Verification items for the finished model (mm, model axes). Face numbers are marked on the shaded views. A direction names the side the tool comes from. Give positions to 0.01 mm unless a question says otherwise; leave off trailing zeros. Loops run counter-clockwise (first coordinate to the right, second up) from the corner with the lowest first, then second, coordinate; pieces in that order, holes last. Notation, with made-up numbers: M 51,37.25 L 92,37.25 A35 ccw 92,70.25 Z; hole C 56.5,31 d1. An arc over 180 degrees is marked long. Answer in a Markdown table with one row per item.
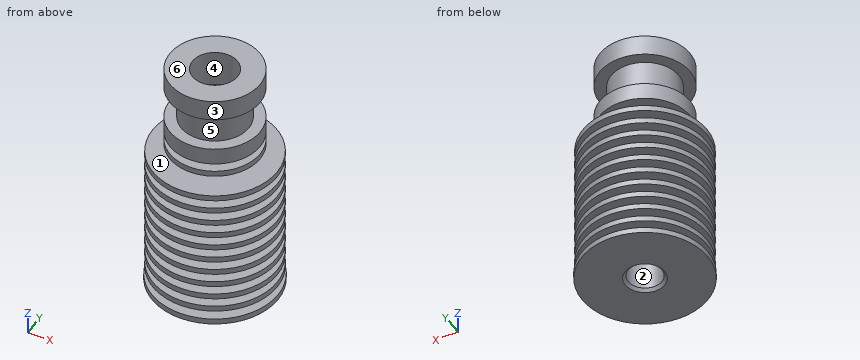
```python
from build123d import *

# Parameters (mm, degrees)
F2_W           = 5
F2_H           = 6
F2_H_2         = 1.5
F4_W           = 8
F4_H           = 1.5
F4_W_2         = 8.1
F4_W_3         = 8.2
F4_W_4         = 8.3
F4_W_5         = 8.4
F4_W_6         = 8.5
F4_W_7         = 8.6
F4_W_8         = 8.7
F4_W_9         = 8.8
F4_W_10        = 8.9
F9_D           = 6
F9_DEPTH       = 10
F9_CSINK_D     = 7
F9_CSINK_ANGLE = 90


with BuildPart() as f1:
    # F0 (on Front) → F1 (revolve)
    with BuildSketch(Plane.XZ):
        Polygon((0, 42.7), (0, 0), (11.15, 0), (11.15, 1), (11, 1), (11, 26), (8, 26), (8, 42.7), align=None)
    revolve(axis=Axis((0, 0, 21.35), (0, 0, 1)))

    # F2 (on Front) → F3 (revolve, cut)
    with BuildSketch(Plane.XZ):
        with Locations((8.5, 36)):
            Rectangle(F2_W, F2_H)
        with Locations((8.5, 29.25)):
            Rectangle(F2_W, F2_H_2)
        with Locations((8.5, 26.75)):
            Rectangle(F2_W, F2_H_2)
    revolve(axis=Axis((0, 0, 22.5), (0, 0, 1)), mode=Mode.SUBTRACT)

    # F4 (on Front) → F5 (revolve, cut)
    with BuildSketch(Plane.XZ):
        with Locations((11, 1.75)):
            Rectangle(F4_W, F4_H)
        with Locations((10.95, 4.25)):
            Rectangle(F4_W_2, F4_H)
        with Locations((10.9, 6.75)):
            Rectangle(F4_W_3, F4_H)
        with Locations((10.85, 9.25)):
            Rectangle(F4_W_4, F4_H)
        with Locations((10.8, 11.75)):
            Rectangle(F4_W_5, F4_H)
        with Locations((10.75, 14.25)):
            Rectangle(F4_W_6, F4_H)
        with Locations((10.7, 16.75)):
            Rectangle(F4_W_7, F4_H)
        with Locations((10.65, 19.25)):
            Rectangle(F4_W_8, F4_H)
        with Locations((10.6, 21.75)):
            Rectangle(F4_W_9, F4_H)
        with Locations((10.55, 24.25)):
            Rectangle(F4_W_10, F4_H)
    revolve(axis=Axis((0, 0, 13.092068), (0, 0, 1)), mode=Mode.SUBTRACT)

    # F6 (on Front) → F7 (revolve, cut)
    with BuildSketch(Plane.XZ):
        Polygon((0, 42.7), (0, 0), (3, 0), (3, 15.1), (2.1, 15.640775), (2.1, 35.058365), (4, 36.2), (4, 42.7), align=None)
    revolve(axis=Axis((0, 0, 21.35), (0, 0, 1)), mode=Mode.SUBTRACT)

    # F9
    with Locations(Plane(origin=(0, 0, 0), x_dir=(1, 0, 0), z_dir=(0, 0, -1))):
        with Locations((0, 0)):
            CounterSinkHole(F9_D / 2, F9_CSINK_D / 2, depth=F9_DEPTH, counter_sink_angle=F9_CSINK_ANGLE)


solid = f1.part
```
Item 1: Sectioned sample at B-B (y = 8.5). State how many separate pieces and enclosed holes the cut face has, and give its area (3 significant figures).
Reported:
| item | result |
|---|---|
| separate pieces | 11 |
| enclosed holes | 0 |
| area | 154 mm^2 |
Item 2: Go/stop test with flat-tipped pins: pin 1 (3 mm diameter, centred on x = -2.5, z = 20, fed in from +Y); pin 2 (1.5 mm diameter, centred on x = -4.5, z = 25.5, fed in from +Y); pin 3 (12 mm diameter, centred on y = 5, z = 32.5, fed in from -X). Record where each tip stops, or that it passes through.
Reported:
| item | result |
|---|---|
| pin 1 | stops at y = 10.95 |
| pin 2 | stops at y = 10.34 |
| pin 3 | stops at x = -8 |
Item 3: Release check for a two-part mould opening along Y. For the marked faces 1, 2 and 3 record: released by +Y, released by -Y, zero draft, split by the parting line, or undercut.
Reported:
| item | result |
|---|---|
| face 1 | zero draft |
| face 2 | undercut |
| face 3 | split by the parting line |
Item 4: Tool access check on the marked faces 4, 5 and 6. Record the directions out of +Z, -Z, +X, -X, +Y, -Y that give a thin tool (end or side, any length) a straight path to the whole face; none if there is none.
Reported:
| item | result |
|---|---|
| face 4 | +Z |
| face 5 | none |
| face 6 | +Z, +X, -X, +Y, -Y |
Item 5: Sectioned sample at A-A (z = 13). Record the cut outline in (x, y), and give its area (3 significant figures).
Reported:
| item | result |
|---|---|
| outline | C 0,0 d22; hole C 0,0 d6 |
| area | 352 mm^2 |
Item 6: Sectioned sample at C-C (z = 37). Record the cut outline in (x, y).
Reported:
| item | result |
|---|---|
| outline | C 0,0 d12; hole C 0,0 d8 |
Item 7: Scan lines: L1, parallel to Y at x = 0, z = 40; L2, parallel to Y at x = 0, z = 26.75; L3, parallel to X at y = 1.75, z = 7. Record each from-to range of solid material in increasing order. Write a range as [from, to].
Reported:
| item | result |
|---|---|
| L1 | y = [-8, -4], [4, 8] |
| L2 | y = [-6, -2.1], [2.1, 6] |
| L3 | x = [-6.57, -2.44], [2.44, 6.57] |
